Build history of the part. All positions in model axes, mm. A direction names the side the tool comes from. Coordinates: 2 decimals unless noted, no trailing zeros. Write each loop counter-clockwise with the first axis right and the second up, starting at its lowest first coordinate (ties: lowest second). Pieces come first, ordered by that corner, then holes.
```python
from build123d import *

# Parameters (mm, degrees)
BOSS_EXTRUDE1_DEPTH = 1.8
BOSS_EXTRUDE4_DEPTH = 8
SKETCH5_W           = 116
SKETCH5_H           = 70
BOSS_EXTRUDE5_DEPTH = 8
SKETCH6_R           = 2.75
CUT_EXTRUDE1_DEPTH  = 123.131240885


with BuildPart() as part:
    # Sketch1 → Boss-Extrude1 (new body)
    with BuildSketch(Plane.XY):
        with BuildLine():
            Line((50, 0), (58, 0))
            Line((58, 0), (58, 80))
            Line((58, 80), (-58, 80))
            Line((-58, 80), (-58, 0))
            Line((-58, 0), (-50, 0))
            ThreePointArc((-50, 0), (0, 50), (50, 0))
        make_face()
    extrude(amount=BOSS_EXTRUDE1_DEPTH)

    # Sketch4 → Boss-Extrude4 (add)
    with BuildSketch(Plane.XY.offset(1.8)):
        with BuildLine():
            Line((-58, 0), (-55, 0))
            ThreePointArc((-55, 0), (0, 55), (55, 0))
            Line((55, 0), (58, 0))
            Line((58, 0), (58, 80))
            Line((58, 80), (-58, 80))
            Line((-58, 80), (-58, 0))
        make_face()
    extrude(amount=BOSS_EXTRUDE4_DEPTH)

    # Sketch5 → Boss-Extrude5 (add)
    with BuildSketch(Plane(origin=(0, 80, 0), x_dir=(1, 0, 0), z_dir=(0, 1, 0))):
        with Locations((0, -44.8)):
            Rectangle(SKETCH5_W, SKETCH5_H)
    extrude(amount=-BOSS_EXTRUDE5_DEPTH)

    # Sketch6 → Cut-Extrude1 (cut, through all)
    with BuildSketch(Plane.XZ.offset(-72)):
        with Locations(Location((-46, 69.8, 0), (0, 0, 270))):
            Circle(SKETCH6_R)
        with Locations(Location((46, 69.8, 0), (0, 0, 270))):
            Circle(SKETCH6_R)
    extrude(amount=-CUT_EXTRUDE1_DEPTH, mode=Mode.SUBTRACT)


solid = part.part
```
1. Flat gauge pins, fed straight in: pin 1 (8 mm diameter, centred on x = -0.5, y = 54.5, fed in from +Z); pin 2 (6.5 mm diameter, centred on x = 46, z = 69.8, fed in from +Y). Where does each tip first touch, or does it go through?
Computed values:
pin 1: stops at z = 9.8
pin 2: stops at y = 80
2. Saw through at D-D on x = 0. List the corners of the cut face in (y, z).
Computed values:
outline: (50, 0) - (80, 0) - (80, 79.8) - (72, 79.8) - (72, 9.8) - (55, 9.8) - (55, 1.8) - (50, 1.8) - close
3. Saw through at B-B on y = 11. List the corners of the cut face in (x, z) (3 decimals), plus the area to 3 significant figures.
Computed values:
outline: (-58, 0) - (-48.775, 0) - (-48.775, 1.8) - (-53.889, 1.8) - (-53.889, 9.8) - (-58, 9.8) - close; (48.775, 0) - (58, 0) - (58, 9.8) - (53.889, 9.8) - (53.889, 1.8) - (48.775, 1.8) - close
area: 99.0 mm2
4. Mould opens along Z. For faces 1 (the face through (47.859, 75.944, 71.827)), 2 (the face through (-45.879, 75.944, 72.547)), 3 (the face through (-4, 50, 1.8)), 4 (the face through (-1, 72, 44)) say: +Z half, -Z half, draft (parallel to the pull), parting line (faces both ways), or undercut.
Computed values:
face 1: undercut
face 2: undercut
face 3: +Z half
face 4: draft
5. Probe line 1 along X through (y, z) = (75.25, 69.8); line 2 along X through (y, z) = (77, 69); line 3 along Y through (x, z) = (40, 30.5). List the from-to ranges inside material, lowest first.
Computed values:
line 1: x = -58 to -48.75, -43.25 to 43.25, 48.75 to 58
line 2: x = -58 to -48.63, -43.37 to 43.37, 48.63 to 58
line 3: y = 72 to 80
6. Saw through at A-A on z = 69.8. List the corners of the cut face in (x, y).
Computed values:
outline: (-58, 72) - (-48.75, 72) - (-48.75, 80) - (-58, 80) - close; (-43.25, 72) - (43.25, 72) - (43.25, 80) - (-43.25, 80) - close; (48.75, 72) - (58, 72) - (58, 80) - (48.75, 80) - close
7. Saw through at C-C on x = 46. List the corners of the cut face in (y, z).
Computed values:
outline: (19.6, 0) - (80, 0) - (80, 67.05) - (72, 67.05) - (72, 9.8) - (30.15, 9.8) - (30.15, 1.8) - (19.6, 1.8) - close; (72, 72.55) - (80, 72.55) - (80, 79.8) - (72, 79.8) - close
8. 3-axis set-ups, long thin cutter, end or side, ignore diameter. For faces 5 (the face through (-1, 61, 9.8)), 6 (the face through (-1.209, 54.987, 5.744)), 7 (the face through (-1, 80, 39)): which of +Z, -Z, +X, -X, +Y, -Y reach the whole face in a straight line?
Computed values:
face 5: +Z, +X, -X, -Y
face 6: +Z, -Y
face 7: +Z, -Z, +X, -X, +Y
